```python
from build123d import *

# Parameters (mm, degrees)
ESBO_O1_W                = 20
ESBO_O1_H                = 25
RESSALTO_EXTRUS_O1_DEPTH = 9
ESBO_O2_R                = 7.5
CORTE_EXTRUS_O1_DEPTH    = 29.390139133
FILETE1_R                = 3
RESSALTO_EXTRUS_O2_DEPTH = 6
RESSALTO_EXTRUS_O3_DEPTH = 6
FILETE3_R                = 1
FILETE5_R                = 3
FILETE6_R                = 1


with BuildPart() as part:
    # Esboço1 → Ressalto-extrusão1 (new body)
    with BuildSketch(Plane(origin=(0, 0, 0), x_dir=(1, 0, 0), z_dir=(0, 1, 0))):
        Rectangle(ESBO_O1_W, ESBO_O1_H)
    extrude(amount=RESSALTO_EXTRUS_O1_DEPTH)

    # Esboço2 → Corte-extrusão1 (cut, through all)
    with BuildSketch(Plane.XY.offset(12.5)):
        with Locations((0, 10)):
            Circle(ESBO_O2_R)
    extrude(amount=-CORTE_EXTRUS_O1_DEPTH, mode=Mode.SUBTRACT)

    # Filete1
    filete1_edges = [part.edges().sort_by_distance(p)[0] for p in [
        (-10, 0, 0),
        (10, 0, 0),
    ]]
    fillet(filete1_edges, radius=FILETE1_R)

    # Esboço3 → Ressalto-extrusão2 (add)
    with BuildSketch(Plane(origin=(0, 9, 0), x_dir=(1, 0, 0), z_dir=(0, 1, 0))):
        Polygon((-16, 10), (-10, 10), (-10, 8.5), (-14, 8.5), (-14, 6.5), (-10, 6.5), (-10, 5), (-16, 5), align=None)
        Polygon((-14, -6.5), (-10, -6.5), (-10, -5), (-16, -5), (-16, -10), (-10, -10), (-10, -8.5), (-14, -8.5), align=None)
    extrude(amount=-RESSALTO_EXTRUS_O2_DEPTH)

    # Esboço4 → Ressalto-extrusão3 (add)
    with BuildSketch(Plane(origin=(0, 9, 0), x_dir=(1, 0, 0), z_dir=(0, 1, 0))):
        Polygon((-16, -10), (-16, -5), (-11, -5), (-11, -6.5), (-14, -6.5), (-14, -8.5), (-11, -8.5), (-11, -10), align=None)
        Polygon((-11, 10), (-16, 10), (-16, 5), (-11, 5), (-11, 6.5), (-14, 6.5), (-14, 8.5), (-11, 8.5), align=None)
    extrude(amount=RESSALTO_EXTRUS_O3_DEPTH)

    # Filete3
    filete3_edges = [part.edges().sort_by_distance(p)[0] for p in [
        (-16, 9, -5),
        (-16, 9, -10),
        (-16, 9, 10),
        (-16, 9, 5),
    ]]
    fillet(filete3_edges, radius=FILETE3_R)

    # Filete5
    # the kernel refuses this fillet: 3 mm, written as the material it adds along each edge
    with BuildSketch(Plane(origin=(-10, 16.5, -5), x_dir=(-1, 0, 0), z_dir=(0, -1, 0))) as filete5_piece_1_section:
        with BuildLine():
            CenterArc((FILETE5_R, -FILETE5_R), FILETE5_R, 90, 90)
            Line((0, -FILETE5_R), (0, 0))
            Line((0, 0), (FILETE5_R, 0))
        make_face()
    filete5_piece_1 = extrude(amount=13.5, mode=Mode.PRIVATE)
    filete5_piece_1 = split(filete5_piece_1, bisect_by=Plane(origin=(-11.589070595, 9, -4.827479681), z_dir=(0, 1, 0)), keep=Keep.TOP, mode=Mode.PRIVATE)
    filete5_piece_1 = split(filete5_piece_1, bisect_by=Plane(origin=(-11, 12, -4.827479681), z_dir=(-1, 0, 0)), keep=Keep.TOP, mode=Mode.PRIVATE)
    filete5_piece_1 = split(filete5_piece_1, bisect_by=Plane(origin=(-11.589070595, 15, -4.827479681), z_dir=(0, -1, 0)), keep=Keep.TOP, mode=Mode.PRIVATE)
    add(filete5_piece_1)
    with BuildSketch(Plane(origin=(-10, 9, -5), x_dir=(-1, 0, 0), z_dir=(0, -1, 0))) as filete5_piece_2_section:
        with BuildLine():
            CenterArc((FILETE5_R, -FILETE5_R), FILETE5_R, 90, 90)
            Line((0, -FILETE5_R), (0, 0))
            Line((0, 0), (FILETE5_R, 0))
        make_face()
    filete5_piece_2 = extrude(amount=6, mode=Mode.PRIVATE)
    filete5_piece_2 = split(filete5_piece_2, bisect_by=Plane(origin=(-11, 6, -4.827479681), z_dir=(-1, 0, 0)), keep=Keep.TOP, mode=Mode.PRIVATE)
    add(filete5_piece_2)
    with BuildSketch(Plane(origin=(-10, 9, -5), x_dir=(-1, 0, 0), z_dir=(0, -1, 0))) as filete5_piece_3_section:
        with BuildLine():
            CenterArc((FILETE5_R, -FILETE5_R), FILETE5_R, 90, 90)
            Line((0, -FILETE5_R), (0, 0))
            Line((0, 0), (FILETE5_R, 0))
        make_face()
    filete5_piece_3 = extrude(amount=6, mode=Mode.PRIVATE)
    filete5_piece_3 = split(filete5_piece_3, bisect_by=Plane(origin=(-11, 6, -4.141402177), z_dir=(1, 0, 0)), keep=Keep.TOP, mode=Mode.PRIVATE)
    add(filete5_piece_3)
    with BuildSketch(Plane(origin=(-10, 16.5, 5), x_dir=(-1, 0, 0), z_dir=(0, -1, 0))) as filete5_piece_4_section:
        with BuildLine():
            CenterArc((FILETE5_R, FILETE5_R), FILETE5_R, 180, 90)
            Line((0, FILETE5_R), (0, 0))
            Line((0, 0), (FILETE5_R, 0))
        make_face()
    filete5_piece_4 = extrude(amount=13.5, mode=Mode.PRIVATE)
    filete5_piece_4 = split(filete5_piece_4, bisect_by=Plane(origin=(-11.589070595, 15, 4.827479681), z_dir=(0, -1, 0)), keep=Keep.TOP, mode=Mode.PRIVATE)
    filete5_piece_4 = split(filete5_piece_4, bisect_by=Plane(origin=(-11.589070595, 9, 4.827479681), z_dir=(0, 1, 0)), keep=Keep.TOP, mode=Mode.PRIVATE)
    filete5_piece_4 = split(filete5_piece_4, bisect_by=Plane(origin=(-11, 12, 4.827479681), z_dir=(-1, 0, 0)), keep=Keep.TOP, mode=Mode.PRIVATE)
    add(filete5_piece_4)
    with BuildSketch(Plane(origin=(-10, 9, 5), x_dir=(-1, 0, 0), z_dir=(0, -1, 0))) as filete5_piece_5_section:
        with BuildLine():
            CenterArc((FILETE5_R, FILETE5_R), FILETE5_R, 180, 90)
            Line((0, FILETE5_R), (0, 0))
            Line((0, 0), (FILETE5_R, 0))
        make_face()
    filete5_piece_5 = extrude(amount=6, mode=Mode.PRIVATE)
    filete5_piece_5 = split(filete5_piece_5, bisect_by=Plane(origin=(-11, 6, 4.827479681), z_dir=(-1, 0, 0)), keep=Keep.TOP, mode=Mode.PRIVATE)
    add(filete5_piece_5)
    with BuildSketch(Plane(origin=(-10, 9, 5), x_dir=(-1, 0, 0), z_dir=(0, -1, 0))) as filete5_piece_6_section:
        with BuildLine():
            CenterArc((FILETE5_R, FILETE5_R), FILETE5_R, 180, 90)
            Line((0, FILETE5_R), (0, 0))
            Line((0, 0), (FILETE5_R, 0))
        make_face()
    filete5_piece_6 = extrude(amount=6, mode=Mode.PRIVATE)
    filete5_piece_6 = split(filete5_piece_6, bisect_by=Plane(origin=(-11, 6, 4.141402177), z_dir=(1, 0, 0)), keep=Keep.TOP, mode=Mode.PRIVATE)
    add(filete5_piece_6)

    # Filete6
    filete6_edges = [part.edges().sort_by_distance(p)[0] for p in [
        (-11, 12, -4.236067977),
        (-11, 12, 4.236067977),
    ]]
    fillet(filete6_edges, radius=FILETE6_R)


solid = part.part
```
For this review, take the finished solid that the model builds, in its own axes (mm). A direction names the side the tool comes from. Coordinates: 2 decimals unless noted, no trailing zeros. Loops run counter-clockwise (first coordinate to the right, second up) from the corner with the lowest first, then second, coordinate; pieces in that order, holes last. Notation, with made-up numbers: (16, -9) - (68, -9) arc R16 cw to (68, -2) - close; hole circle Ø1 at (37.25, 18). An arc over 180 degrees is marked (long way). Use one line per item in the form item = value. Start each with the question number.
1) Take a section at D-D (z = -0.25). State the section outline as (x, y) points, plus the area to 3 significant figures.
2) For pin 1 (2.5 mm diameter, centred on x = -13, y = 6, fed in from -Z); pin 2 (4 mm diameter, centred on x = -4.5, z = -6.5, fed in from +Y); pin 3 (6.5 mm diameter, centred on x = -12.5, z = -4.5, fed in from -Y); pin 4 (1.8 mm diameter, centred on x = -13, z = 7.5, fed in from -Y), all flat-tipped, find the tip position at first contact; note any pin that passes through.
3) To check wall thickness, follow probe 1 along Z at (x, y) = (-13.5, 12.5); probe 2 along Z at (x, y) = (-12, 11.5); probe 3 along X at (y, z) = (8, -8.25). State the ranges of each line that lie inside material, in increasing order. Write a range as from..to.
4) Take a section at B-B (x = -11.5). State the section outline as (y, z) points, plus the area to 3 significant figures.
5) Draft analysis for pull direction X (two halves, no side actions). For faces 1 (the face through (-11, 12, 9)), 2 (the face through (-14, 9, -8)), 3 (the face through (-14.4, 3, 6.8)), state which applies: released by +X, released by -X, zero draft, split by the parting line, or undercut.
6) For faces 4 (the face through (-11, 12, -9)), 5 (the face through (-12, 9, 6.5)), 6 (the face through (-10, 6, -11)), 7 (the face through (-14, 9, -5)), list the 3-axis set-ups (+Z, -Z, +X, -X, +Y, -Y) from which the entire face can be reached by the end or side of a thin tool; tool diameter is ignored.
7) Take a section at A-A (y = 3.75). State how many separate pieces and enclosed holes the cut face has, plus the area to 3 significant figures.
From the geometry:
q1.outline = (-10, 3) arc R3 ccw to (-7, 0) - (7, 0) arc R3 ccw to (10, 3) - (10, 9) - (7.43, 9) arc R7.5 cw to (-7.43, 9) - (-10, 9) - close
q1.area = 103 mm2
q2.pin_1 = -10
q2.pin_2 = 6.26
q2.pin_3 = 1.02
q2.pin_4 = through
q3.probe_1 = -10..-8.5, -6.5..-5, 5..6.5, 8.5..10
q3.probe_2 = -10..-8.5, -6.5..-4.87, 4.87..6.5, 8.5..10
q3.probe_3 = -16..-14, -10..-7.23, 7.23..10
q4.outline = (3, -10) - (15, -10) - (15, -8.5) - (3, -8.5) - close; (3, -6.5) - (15, -6.5) - (15, -5.01) - (9, -5.01) - (9, -4.6) - (3, -4.6) - close; (3, 4.6) - (9, 4.6) - (9, 5.01) - (15, 5.01) - (15, 6.5) - (3, 6.5) - close; (3, 8.5) - (15, 8.5) - (15, 10) - (3, 10) - close
q4.area = 76.7 mm2
q5.face_1 = released by +X
q5.face_2 = undercut
q5.face_3 = zero draft
q6.face_4 = +Z, -Z, +X, +Y
q6.face_5 = +Y, -Y
q6.face_6 = -Z, -X, +Y, -Y
q6.face_7 = -X, +Y, -Y
q7.separate_pieces = 2
q7.enclosed_holes = 2
q7.area = 340 mm2
